```python
from build123d import *

# Parameters (mm, degrees)
F0_R     = 38.1
F1_DEPTH = 76.2
F2_R     = 34.925
F3_DEPTH = 146.05
F4_W     = 3.175
F4_H     = 152.4
F5_DEPTH = 25.4


with BuildPart() as f1:
    # F0 (on Front) → F1 (new body, symmetric)
    with BuildSketch(Plane.XZ):
        Circle(F0_R)
    extrude(amount=F1_DEPTH, both=True)

    # F2 (on face) → F3 (cut)
    with BuildSketch(Plane.XZ.offset(76.2)):
        Circle(F2_R)
    extrude(amount=-F3_DEPTH, mode=Mode.SUBTRACT)

    # F4 (on Top) → F5 (join, symmetric)
    with BuildSketch(Plane.XY):
        with Locations((36.5125, 0)):
            Rectangle(F4_W, F4_H)
    extrude(amount=F5_DEPTH, both=True)


solid = f1.part
```
Verification items for the finished model (mm, model axes). A direction names the side the tool comes from. Coordinates: 2 decimals unless noted, no trailing zeros. Loops run counter-clockwise (first coordinate to the right, second up) from the corner with the lowest first, then second, coordinate; pieces in that order, holes last. Notation, with made-up numbers: (60.25, -30.5) -> (83.25, -30.5) arc R25 ccw to (83.25, -3.5) -> close; hole circle Ø11 at (18, 89.25). An arc over 180 degrees is marked (long way). Put each result on its own line as item: value.
1. Mould release check, pull along X, two halves, no side actions. Record for faces 1 (the face through (0, 69.85, 0)), 2 (the face through (38.1, -1, 0)), 3 (the face through (31, -76.2, -17)): pulls with the +X half, pulls with the -X half, needs draft (parallel to the pull), parting line crosses it, or undercut.
Result set:
face 1: undercut
face 2: pulls with the +X half
face 3: needs draft
2. Section check A-A, the plane y = -60. Record the boundary of the cut face in (x, z) (3 decimals), then the cut area to 3 significant figures.
Result set:
outline: (34.925, -25.4) -> (38.1, -25.4) -> (38.1, 25.4) -> (34.925, 25.4) -> (34.925, 15.227) arc R38.1 ccw (long way) to (34.925, -15.227) -> close; hole circle Ø69.85 at (0, 0)
area: 825 mm^2
3. Tool access check on faces 4 (the face through (36, 1, 25.4)), 5 (the face through (-27.715, -4.197, -21.251)), 6 (the face through (36, 1, -25.4)). Record the directions out of +Z, -Z, +X, -X, +Y, -Y that give a thin tool (end or side, any length) a straight path to the whole face; none if there is none.
Result set:
face 4: +Z, +X, +Y, -Y
face 5: -Y
face 6: -Z, +X, +Y, -Y
4. Section check B-B, the plane x = 0. Record the boundary of the cut face in (y, z) (3 decimals), then the cut area to 3 significant figures.
Result set:
outline: (-76.2, -38.1) -> (76.2, -38.1) -> (76.2, 38.1) -> (-76.2, 38.1) -> (-76.2, 34.925) -> (69.85, 34.925) -> (69.85, -34.925) -> (-76.2, -34.925) -> close
area: 1,410 mm^2
5. Section check D-D, the plane z = 0. Record the boundary of the cut face in (x, y) (3 decimals), then the cut area to 3 significant figures.
Result set:
outline: (-38.1, -76.2) -> (-34.925, -76.2) -> (-34.925, 69.85) -> (34.925, 69.85) -> (34.925, -76.2) -> (38.1, -76.2) -> (38.1, 76.2) -> (-38.1, 76.2) -> close
area: 1,410 mm^2
6. Section check C-C, the plane z = -23.5. Record the boundary of the cut face in (x, y) (3 decimals).
Result set:
outline: (-29.989, -76.2) -> (-25.836, -76.2) -> (-25.836, 69.85) -> (25.836, 69.85) -> (25.836, -76.2) -> (29.989, -76.2) -> (29.989, 76.2) -> (-29.989, 76.2) -> close; (34.925, -76.2) -> (38.1, -76.2) -> (38.1, 76.2) -> (34.925, 76.2) -> close
7. Thickness scan on line 1 (Z direction, x = 0, y = 23) (3 decimals); line 2 (X direction, y = -20.5, z = 18.5) (3 decimals); line 3 (X direction, y = 7.5, z = -25) (3 decimals). Record the ranges inside material, lowest first.
Result set:
line 1: z = -38.1 to -34.925, 34.925 to 38.1
line 2: x = -33.307 to -29.623, 29.623 to 33.307, 34.925 to 38.1
line 3: x = -28.751 to -24.388, 24.388 to 28.751, 34.925 to 38.1
8. Gauge pin test, flat ends, axial feed: P1, Ø5, axis at y = 17.5, z = 18, coming from the -X side; P2, Ø3.5, axis at x = 36.5, y = 24.5, coming from the -Z side; P3, Ø3, axis at x = -14.5, y = -50.5, coming from the -Z side. Record the tip position at first contact, or that the pin passes through.
Result set:
P1: stops at x = -34.8
P2: stops at z = -25.4
P3: stops at z = -35.81
